Autodesk Inventor part; units mm, degrees
ref_plane "Start Plane" through (0, 0, -18.5858) normal (0, 0, 1) x (1, 0, 0)
ref_plane "End Plane" through (0, 0, 618.5525) normal (0, 0, 1) x (1, 0, 0)
ref_plane "Work Plane4" through (-20.7071, 0, 619.2596) normal (0.7071, 0, 0.7071) x (0.7071, 0, -0.7071)
ref_plane "Start Plane" through (0, 0, -18.5858) normal (0, 0, 1) x (1, 0, 0)
ref_plane "End Plane" through (0, 0, 618.5525) normal (0, 0, 1) x (1, 0, 0)
sketch "Sketch" plane through (0, 0, 0) normal (0, 0, 1) x (1, 0, 0)
  line L0 (-20, -14) -> (-20, 14)
  line L1 (-14, 20) -> (14, 20)
  line L2 (20, 14) -> (20, -14)
  line L3 (14, -20) -> (-14, -20)
  arc A0 (-20, -14) -> (-14, -20) centre (-14, -14) ccw
  arc A1 (20, 14) -> (14, 20) centre (14, 14) ccw
  arc A2 (-14, 20) -> (-20, 14) centre (-14, 14) ccw
  arc A3 (14, -20) -> (20, -14) centre (14, -14) ccw
  arc A4 (-14, 17) -> (-17, 14) centre (-14, 14) ccw
  line L4 (-14, 17) -> (14, 17)
  arc A5 (17, 14) -> (14, 17) centre (14, 14) ccw
  line L5 (17, 14) -> (17, -14)
  arc A6 (14, -17) -> (17, -14) centre (14, -14) ccw
  line L6 (14, -17) -> (-14, -17)
  arc A7 (-17, -14) -> (-14, -17) centre (-14, -14) ccw
  line L7 (-17, -14) -> (-17, 14)
  line L8 (0, 29.7397) -> (0, -29.7397) construction
  line L9 (-29.7397, 0) -> (29.7397, 0) construction
  dimension "d7" = 6
  dimension "d9" = 40
  dimension "d11" = 40
  dimension "d12" = 3
  dimension "d15" = 20
  dimension "d16" = 20
extrude "Body" add sketch "Sketch" along normal up to surface (637.1383 mm away) from surface at -18.5858
sketch "Sketch3" plane through (0, 0, 0) normal (0, 0, 1) x (1, 0, 0)
  line L0 (0, 0) -> (10, 0)
ref_plane "Work Plane3" through (0, 0, 0) normal (0, -1, 0) x (1, 0, 0)
ref_plane "Work Plane4" through (-20.7071, 0, 619.2596) normal (0.7071, 0, 0.7071) x (0.7071, 0, -0.7071)
split "Split1" plane through (-20.7071, 0, 619.2596) removes the side toward (0.7071, 0, 0.7071)
ref_plane "Work Plane5" through (-20.7071, 0, -19.2929) normal (0.7071, 0, -0.7071) x (-0.7071, 0, -0.7071)
split "Split2" plane through (-20.7071, 0, -19.2929) removes the side toward (0.7071, 0, -0.7071)
sketch "Sketch4" plane through (0, 0, 0) normal (0, -1, 0) x (1, 0, 0)
  line L0 (-2, -18.5858) -> (12, -18.5858)
  line L1 (-2, 618.5525) -> (12, 618.5525)
  dimension "d18" = 637.1383
equation "\"d7\" = G_IR"
equation "\"d9\" = G_W"
equation "\"d11\" = G_H"
equation "\"d12\" = G_T"
equation "\"d15\" = 0.5 * d9"
equation "\"d16\" = 0.5 * d11"
equation "\"d3\" = G_L"
equation "\"G_W\" = 40"
equation "\"G_H\" = 40"
equation "\"G_T\" = 3"
equation "\"G_IR\" = 6"
equation "\"G_L\" = d18"
equation "\"G_OFFSET_START\" = 18.58579"
equation "\"G_OFFSET_END\" = 18.58579"
equation "\"d13\" = -G_OFFSET_START"
equation "\"d14\" = G_OFFSET_END + B_L"
equation "\"B_L\" = 599.96675"
properties part number "ISO 10799-2 - 40x40x3 - 637,14" material "Steel, Mild"
Verification items for the finished model (mm, model axes). A direction names the side the tool comes from. Coordinates: 2 decimals unless noted, no trailing zeros. Loops run counter-clockwise (first coordinate to the right, second up) from the corner with the lowest first, then second, coordinate; pieces in that order, holes last. Notation, with made-up numbers: (-40, 48) -> (9, 48) arc R33 ccw to (9, 83) -> close; hole circle Ø3 at (1.25, -19.5). An arc over 180 degrees is marked (long way). Answer in a Markdown table with one row per item.
1) Section check C-C (z = 52.5). Record the cut outline in (x, y), and give its area (3 significant figures).
The answers:
| item | result |
|---|---|
| outline | (-20, -14) arc R6 ccw to (-14, -20) -> (14, -20) arc R6 ccw to (20, -14) -> (20, 14) arc R6 ccw to (14, 20) -> (-14, 20) arc R6 ccw to (-20, 14) -> close; hole (-17, -14) arc R3 ccw to (-14, -17) -> (14, -17) arc R3 ccw to (17, -14) -> (17, 14) arc R3 ccw to (14, 17) -> (-14, 17) arc R3 ccw to (-17, 14) -> close |
| area | 421 mm2 |
2) Access from +Z, -Z, +X, -X, +Y, -Y to the whole of each face (thin tool, end or side, straight path). Record for faces 4 (the face through (-20, 0, 296)), 5 (the face through (-17, 0, 296)).
The answers:
| item | result |
|---|---|
| face 4 | +Z, -Z, -X, +Y, -Y |
| face 5 | +Z, -Z |
3) Depth check by flat-ended pin: P1, Ø8, axis at x = -8, y = -11, coming from the +Z side. Enter the tip coordinate at first touch or a pass-through.
The answers:
| item | result |
|---|---|
| P1 | passes through |
4) Draft check along X on faces 1 (the face through (0, 20, 296)), 2 (the face through (17, 0, 296)), 3 (the face through (-0.28, -18.06, 598.83)). Enter one of: released by +X, released by -X, zero draft, split by the parting line, or undercut.
The answers:
| item | result |
|---|---|
| face 1 | zero draft |
| face 2 | undercut |
| face 3 | released by +X |
5) Scan lines: line 1 along Y through (x, z) = (3, 249.5); line 2 along Y through (x, z) = (15, 382). Record each from-to range of solid material in increasing order. Write a range as from..to.
The answers:
| item | result |
|---|---|
| line 1 | y = -20..-17, 17..20 |
| line 2 | y = -19.92..-16.83, 16.83..19.92 |
6) Section check B-B (y = -5). Record the cut outline in (x, z), and give its area (3 significant figures).
The answers:
| item | result |
|---|---|
| outline | (-20, -18.59) -> (-17, -15.59) -> (-17, 615.55) -> (-20, 618.55) -> close; (17, 18.41) -> (20, 21.41) -> (20, 578.55) -> (17, 581.55) -> close |
| area | 3,580 mm2 |
7) Section check A-A (x = -3). Record the cut outline in (y, z).
The answers:
| item | result |
|---|---|
| outline | (-20, -1.59) -> (-17, -1.59) -> (-17, 601.55) -> (-20, 601.55) -> close; (17, -1.59) -> (20, -1.59) -> (20, 601.55) -> (17, 601.55) -> close |
